from build123d import *

# Parameters (mm, degrees)
F1_DEPTH = 5
F3_DEPTH = 5.001
F4_SIZE  = 2
F5_R     = 0.5
F6_R     = 5


with BuildPart() as f1:
    # F0 (on Top) → F1 (new body)
    with BuildSketch(Plane.XY):
        with BuildLine():
            Line((-26.7304610461, 15), (-26.7304610461, 0))
            Line((-26.7304610461, 0), (-26.7304610461, -15))
            Line((-26.7304610461, -15), (33.2695389539, -15))
            ThreePointArc((33.2695389539, -15), (48.2695389539, 0), (33.2695389539, 15))
            Line((33.2695389539, 15), (-26.7304610461, 15))
        make_face()
    extrude(amount=F1_DEPTH)

    # F2 (on face) → F3 (cut, through all)
    with BuildSketch(Plane.XY.offset(5)):
        with BuildLine():
            Line((35.1235885757, -0.75), (48.2507772205, -0.75))
            ThreePointArc((48.2507772205, -0.75), (48.2695389539, 0), (48.2507772205, 0.75))
            Line((48.2507772205, 0.75), (35.1235885757, 0.75))
            ThreePointArc((35.1235885757, 0.75), (35.2327123089, 0.3820345249), (35.2695389539, 0))
            ThreePointArc((35.2695389539, 0), (35.2327123089, -0.3820345249), (35.1235885757, -0.75))
        make_face()
        with BuildLine():
            ThreePointArc((35.1235885757, 0.75), (31.2695389539, 0), (35.1235885757, -0.75))
            Line((35.1235885757, -0.75), (33.2695389539, -0.75))
            Line((33.2695389539, -0.75), (33.2695389539, 0.75))
            Line((33.2695389539, 0.75), (35.1235885757, 0.75))
        make_face()
        with BuildLine():
            Line((33.2695389539, -0.75), (35.1235885757, -0.75))
            ThreePointArc((35.1235885757, -0.75), (35.2327123089, -0.3820345249), (35.2695389539, 0))
            ThreePointArc((35.2695389539, 0), (35.2327123089, 0.3820345249), (35.1235885757, 0.75))
            Line((35.1235885757, 0.75), (33.2695389539, 0.75))
            Line((33.2695389539, 0.75), (33.2695389539, -0.75))
        make_face()
    extrude(amount=-F3_DEPTH, mode=Mode.SUBTRACT)

    # F4
    f4_edges = [f1.edges().sort_by_distance(p)[0] for p in [
        (31.269539, 0, 5),
        (31.269539, 0, 0),
    ]]
    chamfer(f4_edges, length=F4_SIZE)

    # F5
    f5_edges = [f1.edges().sort_by_distance(p)[0] for p in [
        (31.269539, 0, 3),
        (31.269539, 0, 2),
    ]]
    fillet(f5_edges, radius=F5_R)

    # F6
    f6_edges = [f1.edges().sort_by_distance(p)[0] for p in [
        (48.250777, 0.75, 2.5),
        (48.250777, -0.75, 2.5),
    ]]
    fillet(f6_edges, radius=F6_R)


solid = f1.part
Geometry: final body of the model. Coordinates: model frame, mm. A direction names the side the tool comes from. Give positions to 0.01 mm unless a question says otherwise; leave off trailing zeros. Write each loop counter-clockwise with the first axis right and the second up, starting at its lowest first coordinate (ties: lowest second). Pieces come first, ordered by that corner, then holes. Notation, with made-up numbers: (16, 11) - (52, 11) arc R19 ccw to (52, 47) - close; hole circle Ø2 at (27, 45.25). An arc over 180 degrees is marked (long way). Return JSON: item names as keys, results as strings. Group by question number.
1) Set-up query: faces 5 (the conical face through (30.83, 0.1, 3.44)), 6 (the flat face through (39, -0.75, 3)). Return all of +Z, -Z, +X, -X, +Y, -Y with unobstructed straight access to the full face (end or side cutting, diameter ignored); none if empty.
2) Mould query, pull axis X, two halves, no side actions, for faces 1 (the flat face through (-26.73, 0, 2)), 2 (the cylindrical face through (40.09, -13.36, 2.46)), 3 (the conical face through (30.83, 0.1, 1.56)), 4 (the flat face through (3, -15, 2)). Classes: released by +X, released by -X, zero draft, split by the parting line, or undercut.
3) Section C-C on y = 12. Return the cut outline in (x, z).
4) First-contact query: P1, Ø2, axis at x = 36, z = 2, coming from the +Y side; P2, Ø3.5, axis at x = 33.27, y = 0, coming from the -Z side; P3, Ø1.5, axis at y = 7, z = 2, coming from the +X side. Flat tips, straight axial feed; report the tip coordinate or a pass-through.
5) Line query: line 1 (X direction, y = 0, z = 2.75); line 2 (Y direction, x = 42.5, z = 4); line 3 (Y direction, x = 32, z = 2.3). Output: solid intervals per line, ascending.
6) Section B-B on y = -12.25. Return the cut outline in (x, z).
7) Section A-A on z = 4.25. Return the cut outline in (x, y) (3 decimals), plus the area to 3 significant figures.
Filled in:
{
 "1": {"face 5": "+Z", "face 6": "+Z, -Z, +X"},
 "2": {"face 1": "released by -X", "face 2": "released by +X", "face 3": "undercut", "face 4": "zero draft"},
 "3": {"outline": "(-26.73, 0) - (42.27, 0) - (42.27, 5) - (-26.73, 5) - close"},
 "4": {"P1": "stops at y = 14.9", "P2": "passes through", "P3": "stops at x = 46.43"},
 "5": {"line 1": "x = -26.73 to 31.27", "line 2": "y = -11.82 to -0.86, 0.86 to 11.82", "line 3": "y = -15 to -1.55, 1.55 to 15"},
 "6": {"outline": "(-26.73, 0) - (41.93, 0) - (41.93, 5) - (-26.73, 5) - close"},
 "7": {"outline": "(-26.73, -15) - (33.27, -15) arc R15 ccw to (45.542, -8.625) arc R5 ccw to (41.451, -0.75) - (36.432, -0.75) arc R3.25 cw (long way) to (36.432, 0.75) - (41.451, 0.75) arc R5 ccw to (45.542, 8.625) arc R15 ccw to (33.27, 15) - (-26.73, 15) - close", "area": "2,080 mm^2"}
}
